```python
from build123d import *

# Parameters (mm, degrees)
SKETCH1_R               = 3.1623
BOSS_EXTRUDE1_DEPTH     = 11.0998
CUT_EXTRUDE1_DEPTH      = 1
CUT_EXTRUDE1_DEPTH_BACK = 12.0998
SKETCH3_R               = 6.35
BOSS_EXTRUDE2_DEPTH     = 87.122


with BuildPart() as part:
    # Sketch1 → Boss-Extrude1 (new body)
    with BuildSketch(Plane.XY):
        Circle(SKETCH1_R)
    extrude(amount=BOSS_EXTRUDE1_DEPTH)

    # Sketch2 → Cut-Extrude1 (cut, two sides)
    with BuildSketch(Plane(origin=(0, 0, 0), x_dir=(-1, 0, 0), z_dir=(0, 0, -1))) as cut_extrude1_sk:
        Polygon((17.073178183, -20.234228338), (0.001249598, -3.162299753), (-3.162299753, 0.001249598), (-20.234228338, 17.073178183), (-54.378085507, -17.070678986), (-17.070678986, -54.378085507), align=None)
    extrude(amount=CUT_EXTRUDE1_DEPTH, mode=Mode.SUBTRACT)
    extrude(cut_extrude1_sk.sketch, amount=-CUT_EXTRUDE1_DEPTH_BACK, mode=Mode.SUBTRACT)

    # Sketch3 → Boss-Extrude2 (add)
    with BuildSketch(Plane.XY.offset(11.0998)):
        Circle(SKETCH3_R)
    extrude(amount=BOSS_EXTRUDE2_DEPTH)


solid = part.part
```
Can you work these out from the model? Positions are in its coordinate system, mm. Coordinates: 2 decimals unless noted, no trailing zeros. Order: outer loops, then holes, each group sorted by start corner. A loop starts at its lowest first (then second) coordinate and runs counter-clockwise, first axis right, second up.
1. I'm going to push flat-ended pins straight in: pin 1 (5 mm diameter, centred on y = -4, z = 30, fed in from +X); pin 2 (1 mm diameter, centred on y = 4.5, z = 50, fed in from +X). Where does each tip first touch, or does it pass through?
2. If we section it at C-C (y = -2): Please give me the cut outline in (x, z), then the cut area to 3 significant figures.
3. If we section it at A-A (z = 7): Please give me the cut outline in (x, y), then the cut area to 3 significant figures.
4. If we section it at B-B (x = 1.75): Please give me the cut outline in (y, z), then the cut area to 3 significant figures.
5. Thinking about a two-plate mould opening in X: for faces 1 (the face through (1.56, -1.6, 5.47)), 2 (the face through (3, -1, 11.1)), 3 (the face through (-2.16, 2.31, 5.47)), which applies, +X half, -X half, draft (parallel to the pull), parting line (faces both ways), or undercut?
6. I need wall thicknesses on line 1 (Z direction, x = 4.5, y = 0.25); line 2 (Y direction, x = 0.5, z = 52.5); line 3 (Y direction, x = -3.5, z = 12). Which ranges of each line are inside material? Lowest first, please.
7. If we section it at D-D (y = 4.5): Please give me the cut outline in (x, z).
Entries:
1. pin 1: stops at x = 6.17
1. pin 2: stops at x = 4.93
2. outline: (-6.03, 11.1) - (-2.45, 11.1) - (-2.45, 0) - (1.16, 0) - (1.16, 11.1) - (6.03, 11.1) - (6.03, 98.22) - (-6.03, 98.22) - close
2. area: 1,090 mm2
3. outline: (0, -3.16) - (3.16, 0) arc R3.16 ccw (long way) to start
3. area: 28.6 mm2
4. outline: (-6.1, 11.1) - (-1.41, 11.1) - (-1.41, 0) - (2.63, 0) - (2.63, 11.1) - (6.1, 11.1) - (6.1, 98.22) - (-6.1, 98.22) - close
4. area: 1,110 mm2
5. face 1: +X half
5. face 2: draft
5. face 3: parting line
6. line 1: z = 11.1 to 98.22
6. line 2: y = -6.33 to 6.33
6. line 3: y = -5.3 to 5.3
7. outline: (-4.48, 11.1) - (4.48, 11.1) - (4.48, 98.22) - (-4.48, 98.22) - close
